Design review of the part built by this model. Coordinates are the model's own, in mm. Face numbers are marked on the shaded views. Round coordinates to 2 decimals unless told otherwise and drop trailing zeros. Use a Markdown table: item, result.
from build123d import *

# Parameters (mm, degrees)
SKETCH18_W          = 20
SKETCH18_H          = 12
BOSS_EXTRUDE2_DEPTH = 10
SKETCH19_R          = 1.5
CUT_EXTRUDE1_DEPTH  = 15
SWEEP2_PROFILE_R    = 5
SKETCH39_R          = 39
SKETCH39_R_2        = 37
BOSS_EXTRUDE4_DEPTH = 50


with BuildPart() as part:
    # Sketch1 → Revolve6 (revolve)
    with BuildSketch(Plane(origin=(0, 0, 0), x_dir=(0, 0, -1), z_dir=(1, 0, 0))):
        with BuildLine():
            Line((0, 37), (0, 42))
            add(Edge.make_bspline(
                [(0, 42), (92.195444573, 42), (200, 0)],
                knots=[0, 0, 0, 1, 1, 1], degree=2))
            Line((200, 0), (198, 0))
            add(Edge.make_bspline(
                [(0, 37), (91.00549434, 37), (198, 0)],
                knots=[0, 0, 0, 1, 1, 1], degree=2))
        make_face()
    revolve(axis=Axis((0, 0, 198), (0, 0, -1)))



with BuildPart() as body_2:
    # Sketch15 → Revolve7 (revolve)
    with BuildSketch(Plane(origin=(0, 0, 0), x_dir=(0, 0, -1), z_dir=(1, 0, 0))):
        with BuildLine():
            Line((0, 37), (0, 0))
            Line((0, 0), (198, 0))
            add(Edge.make_bspline(
                [(0, 37), (91.00549434, 37), (198, 0)],
                knots=[0, 0, 0, 1, 1, 1], degree=2))
        make_face()
    revolve(axis=Axis((0, 0, -198), (0, 0, 1)))

    # Sketch16 → Cut-Revolve1 (revolve, cut)
    with BuildSketch(Plane(origin=(0, 0, 0), x_dir=(0, 0, -1), z_dir=(1, 0, 0))):
        with BuildLine():
            Line((85, 1.5e-08), (0, 0))
            Line((0, 0), (2.5e-08, 37))
            add(Edge.make_bspline(
                [(2.5e-08, 37), (40.886337168, 36.999999998), (85, 29.531680157)],
                knots=[0, 0, 0, 1, 1, 1], degree=2))
            Line((85, 29.531680157), (85, 1.5e-08))
        make_face()
    revolve(axis=Axis((0, 1.5e-08, -85), (0, -1.7796762949934384e-10, 1.0)), mode=Mode.SUBTRACT)


with BuildPart() as part_1:
    add(part.part)

    add(body_2.part)  # Boss-Extrude2 merges body 2
    # Sketch18 → Boss-Extrude2 (add)
    with BuildSketch(Plane.XY.offset(-85.000000003)):
        with Locations((0, 18)):
            Rectangle(SKETCH18_W, SKETCH18_H)
        with Locations((0, -18)):
            Rectangle(SKETCH18_W, SKETCH18_H)
    extrude(amount=BOSS_EXTRUDE2_DEPTH)

    # Sketch19 → Cut-Extrude1 (cut)
    with BuildSketch(Plane.XY.offset(-75.000000003)):
        with Locations(Location((-8, 18, 0), (0, 0, 270))):
            Circle(SKETCH19_R)
        with Locations(Location((8, 18, 0), (0, 0, 270))):
            Circle(SKETCH19_R)
        with Locations(Location((-8, -18, 0), (0, 0, 270))):
            Circle(SKETCH19_R)
        with Locations(Location((8, -18, 0), (0, 0, 270))):
            Circle(SKETCH19_R)
    extrude(amount=-CUT_EXTRUDE1_DEPTH, mode=Mode.SUBTRACT)

    # Sweep2: sweep along a path in Sketch22
    with BuildLine(Plane(origin=(0, 0, 0), x_dir=(0, 0, -1), z_dir=(1, 0, 0))) as sweep2_path:
        ThreePointArc((74.999999999, 18.000000013), (59.443329555, -3e-09), (75.000000005, -18.000000014))
    # Sweep2 profile (on start of the path) → Sweep2 (sweep)
    with BuildSketch(Plane(origin=(0, 18.000000013, -74.999999999), x_dir=(0, 0.9894527315338124, 0.14485610812208577), z_dir=(0, -0.14485610812208577, 0.9894527315338124))):
        Circle(SWEEP2_PROFILE_R)
    sweep(path=sweep2_path.line)

    # Sketch39 → Boss-Extrude4 (add)
    with BuildSketch(Plane.XY):
        Circle(SKETCH39_R)
        Circle(SKETCH39_R_2, mode=Mode.SUBTRACT)
    extrude(amount=BOSS_EXTRUDE4_DEPTH)


solid = part_1.part
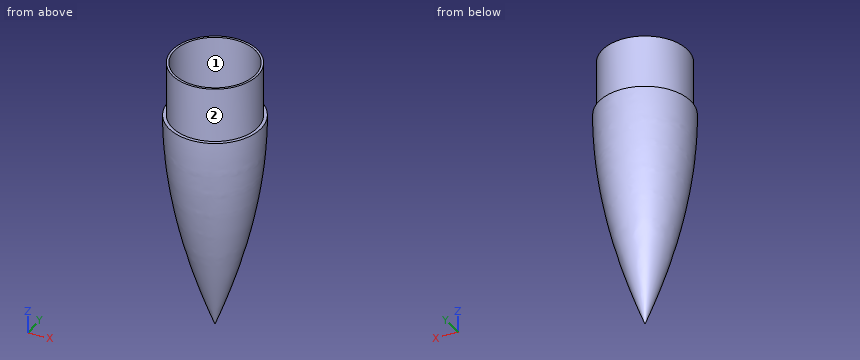
1. Wall thickness on line 1 along X through (y, z) = (-18, -80.75); line 2 along X through (y, z) = (-18, -78); line 3 along Y through (x, z) = (-27, -69): over which ranges is each line inside the solid? List them lowest first. Write a range as from..to.
Check values:
| item | result |
|---|---|
| line 1 | x = -29.42..-24.29, -10..-9.5, -6.5..6.5, 9.5..10, 24.29..29.42 |
| line 2 | x = -29.99..-24.84, -10..-9.5, -6.5..6.5, 9.5..10, 24.84..29.99 |
| line 3 | y = -24.51..-17.19, 17.19..24.51 |
2. The part is to be moulded in two halves that separate along X. For the marked faces 1 and 2, say which applies: pulls with the +X half, pulls with the -X half, needs draft (parallel to the pull), parting line crosses it, or undercut.
Check values:
| item | result |
|---|---|
| face 1 | undercut |
| face 2 | parting line crosses it |
3. Insertion check: pin 1 (10 mm diameter, centred on y = -6, z = -159, fed in from -X); pin 2 (8 mm diameter, centred on y = 2.5, z = -172.5, fed in from +X); pin 3 (5 mm diameter, centred on x = -8, y = -18, fed in from +Z); pin 4 (1 mm diameter, centred on x = 29, y = -33, fed in from +Z). Each pin has a flat end and moves straight along its axis. Give the tip position at first contact, or say it passes through.
Check values:
| item | result |
|---|---|
| pin 1 | stops at x = -15.64 |
| pin 2 | stops at x = 11.35 |
| pin 3 | stops at z = -75 |
| pin 4 | passes through |
